```python
from build123d import *
from build123d.topology import SkipClean

# Parameters (mm, degrees)
SKETCH1_R          = 105.6
EXTRUDE1_DEPTH     = 5
SKETCH2_R          = 1.5875
CUT_EXTRUDE1_DEPTH = 6
EXTRUDE2_DEPTH     = 10
CIRPATTERN1_COUNT  = 3
EXTRUDE3_DEPTH     = 10
EXTRUDE4_DEPTH     = 8
FILLET1_R          = 1


with BuildPart() as part:
    # Sketch1 → Extrude1 (new body)
    with BuildSketch(Plane(origin=(0, 0, 0), x_dir=(1, 0, 0), z_dir=(0, 1, 0))):
        with Locations(Location((0, 0, 0), (0, 0, 270))):  # turned: the seam where the file's is
            Circle(SKETCH1_R)
    extrude(amount=EXTRUDE1_DEPTH)

    # Sketch2 → Cut-Extrude1 (cut, through all)
    with BuildSketch(Plane(origin=(0, 5, 0), x_dir=(1, 0, 0), z_dir=(0, 1, 0))):
        with Locations(Location((-62.980195842, 77.675574872, 0), (0, 0, 270))):  # turned: the seam where the file's is
            Circle(SKETCH2_R)
        with Locations(Location((62.980195842, -77.675574872, 0), (0, 0, 270))):  # turned: the seam where the file's is
            Circle(SKETCH2_R)
    extrude(amount=-CUT_EXTRUDE1_DEPTH, mode=Mode.SUBTRACT)

    # Sketch3 → Extrude2 (add)
    with BuildSketch(Plane.XZ):
        with BuildLine():
            Line((-25, 102.598050664), (-25, 98.579358894))
            ThreePointArc((-25, 98.579358894), (0, 101.7), (25, 98.579358894))
            Line((25, 98.579358894), (25, 102.598050664))
            ThreePointArc((25, 102.598050664), (0, 105.6), (-25, 102.598050664))
        make_face()
    extrude2 = extrude(amount=EXTRUDE2_DEPTH)

    # CirPattern1: Extrude2 ×3 about axis
    with SkipClean():  # keep this step's faces unmerged: merging them makes the solid invalid here
        cirpattern1_axis = Axis((0, 0, 0), (0, 1, 0))
        for i in range(1, CIRPATTERN1_COUNT):
            add(extrude2.rotate(cirpattern1_axis, i * 360 / CIRPATTERN1_COUNT))

    # Sketch4 → Extrude3 (cut)
    with SkipClean():  # keep this step's faces unmerged: merging them makes the solid invalid here
        with BuildSketch(Plane.XZ.offset(10)):
            with BuildLine():
                Line((5.5, 105.456673568), (5.5, 101.551169368))
                ThreePointArc((5.5, 101.551169368), (0, 101.7), (-5.5, 101.551169368))
                Line((-5.5, 101.551169368), (-5.5, 105.456673568))
                ThreePointArc((-5.5, 105.456673568), (0, 105.6), (5.5, 105.456673568))
            make_face()
        extrude(amount=-EXTRUDE3_DEPTH, mode=Mode.SUBTRACT)

    # Sketch5 → Extrude4 (cut)
    with SkipClean():  # keep this step's faces unmerged: merging them makes the solid invalid here
        with BuildSketch(Plane.XZ.offset(10)):
            with BuildLine():
                Line((72.872229091, -70.940314542), (76.352518254, -72.949660426))
                ThreePointArc((76.352518254, -72.949660426), (91.45228264, -52.8), (101.352518254, -29.648390237))
                Line((101.352518254, -29.648390237), (97.872229091, -27.639044353))
                ThreePointArc((97.872229091, -27.639044353), (88.074783565, -50.85), (72.872229091, -70.940314542))
            make_face()
            with BuildLine():
                Line((-76.352518254, -72.949660426), (-72.872229091, -70.940314542))
                ThreePointArc((-72.872229091, -70.940314542), (-88.074783565, -50.85), (-97.872229091, -27.639044353))
                Line((-97.872229091, -27.639044353), (-101.352518254, -29.648390237))
                ThreePointArc((-101.352518254, -29.648390237), (-91.45228264, -52.8), (-76.352518254, -72.949660426))
            make_face()
        extrude(amount=-EXTRUDE4_DEPTH, mode=Mode.SUBTRACT)

    # Fillet1
    fillet1_edges = [part.edges().sort_by_distance(p)[0] for p in [
        (25, -10, 100.588704779),
        (5.5, -10, 103.503921468),
        (-5.5, -10, 103.503921468),
        (-25, -10, 100.588704779),
        (99.612373672, -2, -28.643717295),
        (74.612373672, -2, -71.944987484),
        (-74.612373672, -2, -71.944987484),
        (-99.612373672, -2, -28.643717295),
    ]]
    fillet(fillet1_edges, radius=FILLET1_R)


solid = part.part
```
For this review, take the finished solid that the model builds, in its own axes (mm). A direction names the side the tool comes from. Give positions to 0.01 mm unless a question says otherwise; leave off trailing zeros. Write each loop counter-clockwise with the first axis right and the second up, starting at its lowest first coordinate (ties: lowest second). Pieces come first, ordered by that corner, then holes. Notation, with made-up numbers: M -3.5,28.5 L 43.5,28.5 A25 ccw 43.5,49.5 Z; hole C 33.25,54 d9. An arc over 180 degrees is marked long. One line per item, written item: value.
1) The part is to be moulded in two halves that separate along X. For faces 4 (the cylindrical face through (-15.46, -4.93, 100.52)), 5 (the flat face through (15, -10, 102)), say which applies: +X half, -X half, draft (parallel to the pull), parting line (faces both ways), or undercut.
Results are:
face 4: undercut
face 5: draft
2) For P1, Ø4.5, axis at y = -5, z = 101, coming from the -X side; P2, Ø4, axis at x = -49.5, z = 25, coming from the -Y side; P3, Ø22, axis at x = 91, z = -53, coming from the -Y side, all flat-tipped, find the tip position at first contact; note any pin that passes through.
Results are:
P1: stops at x = -25
P2: stops at y = 0
P3: stops at y = -2
3) Take a section at B-B, the plane x = 0. Write out the cut boundary in (y, z).
Results are:
outline: M 0,-105.6 L 5,-105.6 L 5,105.6 L 0,105.6 Z
4) Take a section at D-D, the plane x = -89. Write out the cut boundary in (y, z), then the cut area to 3 significant figures.
Results are:
outline: M -2,-56.84 L 5,-56.84 L 5,56.84 L 0,56.84 L 0,-49.21 L -2,-49.21 Z
area: 584 mm²
5) Take a section at C-C, the plane z = 0. Write out the cut boundary in (x, y).
Results are:
outline: M -105.6,0 L 105.6,0 L 105.6,5 L -105.6,5 Z
6) Take a section at A-A, the plane y = -6.5. Write out the cut boundary in (x, z).
Results are:
outline: M -25,98.58 A101.7 cw -5.5,101.55 L -5.5,105.46 A105.6 ccw -25,102.6 Z; M 5.5,101.55 A101.7 cw 25,98.58 L 25,102.6 A105.6 ccw 5.5,105.46 Z
7) For faces 1 (the cylindrical face through (-87.897, -0.986, -51.156)), 2 (the flat face through (-89, -2, -50)), 3 (the cylindrical face through (15.19, -4.93, 100.56)), list the 3-axis set-ups (+Z, -Z, +X, -X, +Y, -Y) from which the entire face can be reached by the end or side of a thin tool; tool diameter is ignored.
Results are:
face 1: +Z, -Y
face 2: +Z, -Z, +X, -X, -Y
face 3: -Z, -Y
8) For line 1 (Y direction, x = -93, z = -31); line 2 (Z direction, x = -18.5, y = -3.25); line 3 (Z direction, x = -28, y = 1.25), list the stretches that pass through material, from the lowest coordinate up. Write a range as from..to.
Results are:
line 1: y = 0..5
line 2: z = 100..103.97
line 3: z = -101.82..101.82
